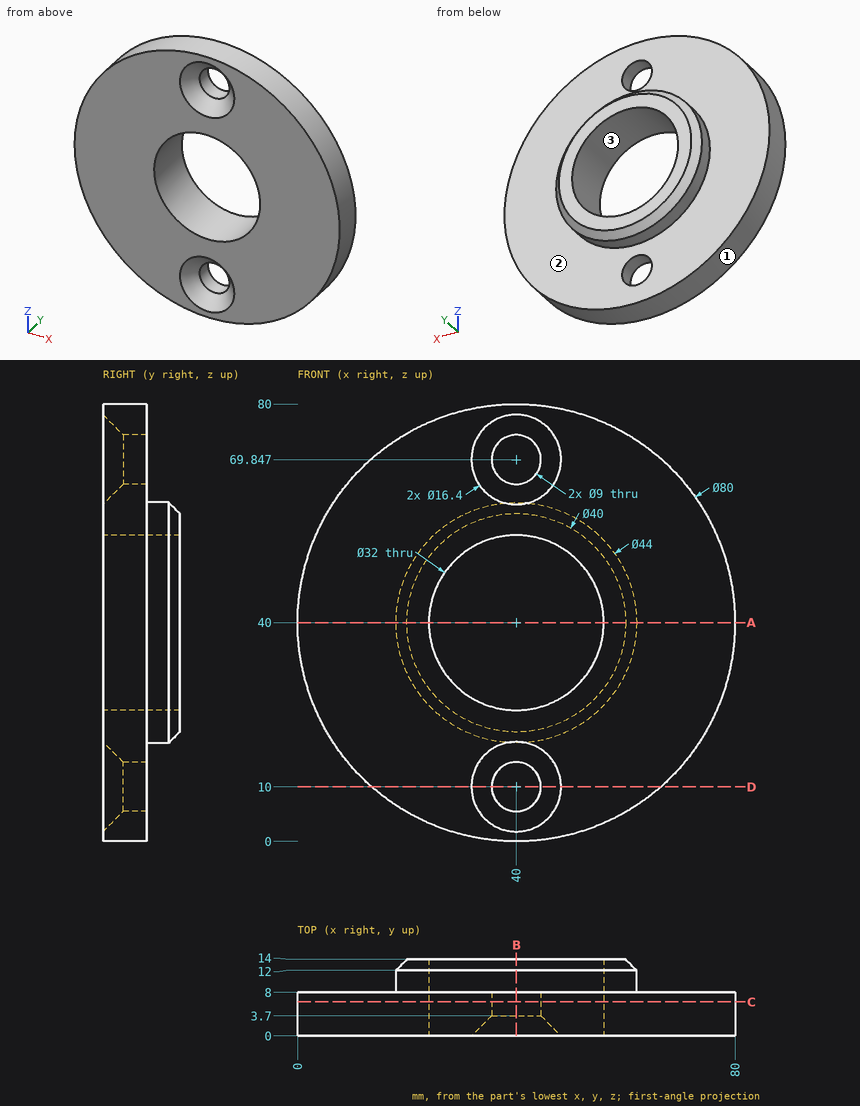
Geometry check sheet. Reference: drawing and pictorial views, mm from the part's lowest x, y, z. Give positions to 0.01 mm unless a question says otherwise; leave off trailing zeros. Write each loop counter-clockwise with the first axis right and the second up, starting at its lowest first coordinate (ties: lowest second). Pieces come first, ordered by that corner, then holes.
Item 1: Draft check along X on the marked faces 1, 2 and 3. Enter one of: released by +X, released by -X, zero draft, split by the parting line, or undercut.
Item 2: Cross-section at C-C (y = 6.25). Enter the section's corners in (x, z).
Item 3: Cross-section at A-A (z = 40). Enter the section's corners in (x, y).
Item 4: Cross-section at D-D (z = 10). Enter the section's corners in (x, y).
Item 5: Scan lines: L1, parallel to Z at x = 40, y = 5.65; L2, parallel to Z at x = 39.5, y = 10.5; L3, parallel to Z at x = 37, y = 5.75 (1 decimal). Record each from-to range of solid material in increasing order.
Item 6: Gauge pin test, flat ends, axial feed: pin 1 (2 mm diameter, centred on y = 4.5, z = 52.5, fed in from -X); pin 2 (1.5 mm diameter, centred on x = 63, y = 7.5, fed in from -Z); pin 3 (4 mm diameter, centred on x = 17.5, y = 9.5, fed in from +Z) (1 decimal). Record the tip position at first contact, or that the pin passes through.
Item 7: Cross-section at B-B (x = 40). Enter the section's corners in (y, z), and give its area (3 significant figures).
Report:
1. face 1: split by the parting line
1. face 2: zero draft
1. face 3: undercut
2. outline: circle Ø80 at (40, 40); hole circle Ø32 at (40, 40); hole circle Ø9 at (40, 10); hole circle Ø9 at (40, 69.85)
3. outline: (0, 0) - (24, 0) - (24, 14) - (20, 14) - (18, 12) - (18, 8) - (0, 8) - close; (56, 0) - (80, 0) - (80, 8) - (62, 8) - (62, 12) - (60, 14) - (56, 14) - close
4. outline: (13.54, 0) - (31.8, 0) - (35.5, 3.7) - (35.5, 8) - (13.54, 8) - close; (44.5, 3.7) - (48.2, 0) - (66.46, 0) - (66.46, 8) - (44.5, 8) - close
5. L1: z = 0 to 5.5, 14.5 to 24, 56 to 65.35, 74.35 to 80
5. L2: z = 18.01 to 24.01, 55.99 to 61.99
5. L3: z = 0.1 to 6.6, 13.4 to 24.3, 55.7 to 66.5, 73.2 to 79.9
6. pin 1: stops at x = 1.69
6. pin 2: stops at z = 6.76
6. pin 3: stops at z = 73.9
7. outline: (0, 0) - (8, 0) - (8, 5.5) - (3.7, 5.5) - (0, 1.8) - close; (0, 18.2) - (3.7, 14.5) - (8, 14.5) - (8, 18) - (12, 18) - (14, 20) - (14, 24) - (0, 24) - close; (0, 56) - (14, 56) - (14, 60) - (12, 62) - (8, 62) - (8, 65.35) - (3.7, 65.35) - (0, 61.65) - close; (0, 78.05) - (3.7, 74.35) - (8, 74.35) - (8, 80) - (0, 80) - close
7. area: 281 mm2
